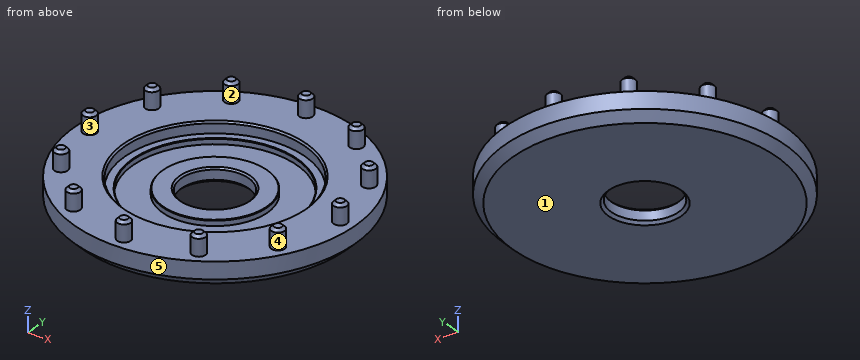
from build123d import *

# Parameters (mm, degrees)
SKETCH1_R                    = 50
BOSS_EXTRUDE1_DEPTH          = 9
SKETCH2_R                    = 2.4
BOSS_EXTRUDE2_DEPTH          = 7
CHAMFER1_SIZE                = 1
CIRPATTERN1_COUNT            = 12
CHAMFER1_OF_CIRPATTERN1_SIZE = 1
SKETCH3_R                    = 32.15
CUT_EXTRUDE1_DEPTH           = 4
SKETCH4_R                    = 12
CUT_EXTRUDE2_DEPTH           = 72.281133549
CHAMFER2_SIZE                = 0.6
SKETCH5_R                    = 29.3
SKETCH5_R_2                  = 18.7
CUT_EXTRUDE3_DEPTH           = 2
CHAMFER3_SIZE                = 0.2
CHAMFER4_SIZE                = 3
CHAMFER5_SIZE                = 1
CHAMFER6_SIZE                = 0.6
SCALE1_SCALE                 = 0.4


with BuildPart() as part:
    # Sketch1 → Boss-Extrude1 (new body)
    with BuildSketch(Plane.XY):
        Circle(SKETCH1_R)
    extrude(amount=-BOSS_EXTRUDE1_DEPTH)

    # Sketch2 → Boss-Extrude2 (add)
    with BuildSketch(Plane.XY):
        with Locations((45, 0)):
            Circle(SKETCH2_R)
    boss_extrude2 = extrude(amount=BOSS_EXTRUDE2_DEPTH)

    # Chamfer1
    chamfer1_edges = [part.edges().sort_by_distance(p)[0] for p in [
        (42.6, 0, 7),
    ]]
    chamfer(chamfer1_edges, length=CHAMFER1_SIZE)

    # CirPattern1: Boss-Extrude2 ×12 about axis
    cirpattern1_axis = Axis((0, 0, 0), (0, 0, 1))
    for i in range(1, CIRPATTERN1_COUNT):
        add(boss_extrude2.rotate(cirpattern1_axis, i * 360 / CIRPATTERN1_COUNT))

    # Chamfer1 of CirPattern1
    chamfer1_of_cirpattern1_edges = [part.edges().sort_by_distance(p)[0] for p in [
        (36.892682201, 21.3, 7),
        (21.3, 36.892682201, 7),
        (0, 42.6, 7),
        (-21.3, 36.892682201, 7),
        (-36.892682201, 21.3, 7),
        (-42.6, 0, 7),
        (-36.892682201, -21.3, 7),
        (-21.3, -36.892682201, 7),
        (0, -42.6, 7),
        (21.3, -36.892682201, 7),
        (36.892682201, -21.3, 7),
    ]]
    chamfer(chamfer1_of_cirpattern1_edges, length=CHAMFER1_OF_CIRPATTERN1_SIZE)

    # Sketch3 → Cut-Extrude1 (cut)
    with BuildSketch(Plane.XY):
        Circle(SKETCH3_R)
    extrude(amount=-CUT_EXTRUDE1_DEPTH, mode=Mode.SUBTRACT)

    # Sketch4 → Cut-Extrude2 (cut, through all)
    with BuildSketch(Plane.XY):
        Circle(SKETCH4_R)
    extrude(amount=-CUT_EXTRUDE2_DEPTH, mode=Mode.SUBTRACT)

    # Chamfer2
    chamfer2_edges = [part.edges().sort_by_distance(p)[0] for p in [
        (-32.15, 0, 0),
    ]]
    chamfer(chamfer2_edges, length=CHAMFER2_SIZE)

    # Sketch5 → Cut-Extrude3 (cut)
    with BuildSketch(Plane.XY.offset(-4)):
        Circle(SKETCH5_R)
        Circle(SKETCH5_R_2, mode=Mode.SUBTRACT)
    extrude(amount=-CUT_EXTRUDE3_DEPTH, mode=Mode.SUBTRACT)

    # Chamfer3
    chamfer3_edges = [part.edges().sort_by_distance(p)[0] for p in [
        (-29.3, 0, -4),
        (-18.7, 0, -4),
    ]]
    chamfer(chamfer3_edges, length=CHAMFER3_SIZE)

    # Chamfer4
    chamfer4_edges = [part.edges().sort_by_distance(p)[0] for p in [
        (-50, 0, -9),
    ]]
    chamfer(chamfer4_edges, length=CHAMFER4_SIZE)

    # Chamfer5
    chamfer5_edges = [part.edges().sort_by_distance(p)[0] for p in [
        (-12, 0, -9),
    ]]
    chamfer(chamfer5_edges, length=CHAMFER5_SIZE)

    # Chamfer6
    chamfer6_edges = [part.edges().sort_by_distance(p)[0] for p in [
        (-12, 0, -4),
    ]]
    chamfer(chamfer6_edges, length=CHAMFER6_SIZE)


with BuildPart() as part_1:
    # Scale1: scaled about (0, 0, -4.695771531)
    add(part.part.scale(SCALE1_SCALE).moved(Location((0, 0, -2.817462919))))


solid = part_1.part
Could you check a few things on this model? Use its own coordinates, in mm. Face numbers are marked on the shaded views. A direction names the side the tool comes from. Give positions to 0.01 mm unless a question says otherwise; leave off trailing zeros. Answer in a Markdown table with one row per item. Add a question column.
Item 1: For the marked faces 4 and 5, which set-ups out of +Z, -Z, +X, -X, +Y, -Y let a thin tool reach every point of the face, with its end or its side?
Item 2: We'd pull the mould along Y, two halves only. Please class the marked faces 1, 2 and 3: pulls with the +Y half, pulls with the -Y half, needs draft (parallel to the pull), parting line crosses it, or undercut.
Item 3: I'm going to push flat-ended pins straight in: P1, Ø2, axis at x = -4.5, z = -4.5, coming from the +Y side; P2, Ø1, axis at x = -13.5, z = -2, coming from the -Y side; P3, Ø8, axis at x = 1.5, y = -8.5, coming from the +Z side; P4, Ø2, axis at x = -16, z = -3.5, coming from the +Y side. Where does each tip first touch, or does it pass through?
Item 4: Please list where these lines run through material, in increasing order: probe 1 along Y at (x, z) = (0, -4.95); probe 2 along Y at (x, z) = (0, -3.35); probe 3 along Z at (x, y) = (-6.5, 4).
Result:
| question | item | result |
|---|---|---|
| 1 | face 4 | +Z |
| 1 | face 5 | +Z, -Z |
| 2 | face 1 | needs draft |
| 2 | face 2 | undercut |
| 2 | face 3 | parting line crosses it |
| 3 | P1 | y = 19.69 |
| 3 | P2 | through |
| 3 | P3 | z = -4.42 |
| 3 | P4 | y = 13.23 |
| 4 | probe 1 | -20 to -11.72, -7.48 to -4.8, 4.8 to 7.48, 11.72 to 20 |
| 4 | probe 2 | -20 to -12.86, 12.86 to 20 |
| 4 | probe 3 | -6.42 to -5.22 |
